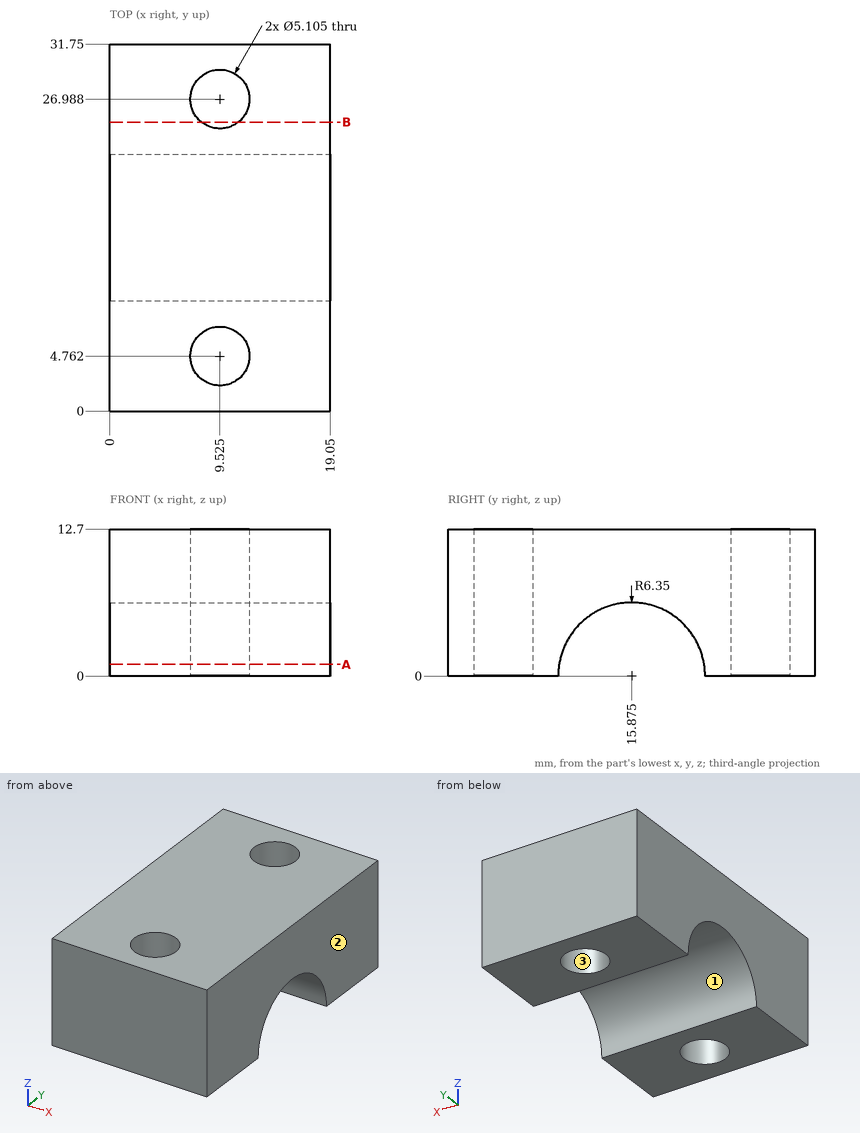
Design review of the part shown in the three views and the two pictorial views. Dimensions are in mm from the part's minimum x, y and z. Coordinates: 2 decimals unless noted, no trailing zeros. Loops run counter-clockwise (first coordinate to the right, second up) from the corner with the lowest first, then second, coordinate; pieces in that order, holes last.
Q1. We need section A-A on z = 1. State how many separate pieces and enclosed holes the cut face has, and give its area (3 significant figures).
Reported:
separate pieces: 2
enclosed holes: 2
area: 325 mm2
Q2. To check wall thickness, follow line 1 (X direction, y = 5, z = 5.75); line 2 (X direction, y = 28, z = 5.5); line 3 (Y direction, x = 2.25, z = 2). State the ranges of each line that lie inside material, in increasing order.
Reported:
line 1: x = 0 to 6.98, 12.07 to 19.05
line 2: x = 0 to 7.18, 11.87 to 19.05
line 3: y = 0 to 9.85, 21.9 to 31.75
Q3. For pin 1 (1.5 mm diameter, centred on x = 5.5, y = 16.5, fed in from -Z); pin 2 (1.5 mm diameter, centred on x = 12, y = 13.5, fed in from -Z), all flat-tipped, find the tip position at first contact; note any pin that passes through.
Reported:
pin 1: stops at z = 6.2
pin 2: stops at z = 5.53
Q4. The part is to be moulded in two halves that separate along X. For the marked faces 1, 2 and 3, say which applies: +X half, -X half, draft (parallel to the pull), parting line (faces both ways), or undercut.
Reported:
face 1: draft
face 2: +X half
face 3: undercut
Q5. We need section B-B on y = 25. State the section outline as (x, z) points.
Reported:
outline: (0, 0) - (7.92, 0) - (7.92, 12.7) - (0, 12.7) - close; (11.13, 0) - (19.05, 0) - (19.05, 12.7) - (11.13, 12.7) - close
